Here's how the part is built. I have some questions about the finished solid (model axes, mm). A direction names the side the tool comes from. Round coordinates to 2 decimals unless told otherwise and drop trailing zeros. Order: outer loops, then holes, each group sorted by start corner. A loop starts at its lowest first (then second) coordinate and runs counter-clockwise, first axis right, second up. Notation, with made-up numbers: (-10, 87.25) -> (2, 87.25) arc R33 ccw to (2, 121.25) -> close; hole circle Ø6 at (68, 77). An arc over 180 degrees is marked (long way). Use a Markdown table: item, result. Add a question column.
(1) I want a section at D-D, the plane x = -8. Please give me the cut outline in (y, z), then the cut area to 3 significant figures.
(2) I'm going to push flat-ended pins straight in: P1, Ø12.5, axis at x = 2, z = 16.5, coming from the -Y side; P2, Ø11, axis at x = 1, z = 14.5, coming from the -Y side; P3, Ø5, axis at x = -8, y = -22, coming from the +Z side. Where does each tip first touch, or does it pass through?
(3) I want a section at C-C, the plane z = 13.5. Please give me the cut outline in (x, y).
(4) If I drill on probe 1 along Z at (x, y) = (0, 1.1); probe 2 along Z at (x, y) = (0, 8.55); probe 3 along Y at (x, z) = (8.5, 0.5), over which ranges is the centre line in solid material (lowest first)?
(5) Thinking about a two-plate mould opening in X: for faces 1 (the face through (-12.7, 0.5, -1.8)), 2 (the face through (2, 5.08, 26)), 3 (the face through (0, 10.16, 5)), which applies, pulls with the +X half, pulls with the -X half, needs draft (parallel to the pull), parting line crosses it, or undercut?
(6) I want a section at A-A, the plane z = 27.94. Please give me the cut outline in (x, y), then the cut area to 3 significant figures.
(7) I want a section at B-B, the plane x = 0.5. Please give me the cut outline in (y, z).
(8) On a 3-axis mill with a long thin cutter (end or side, diameter ignored), from which of +Z, -Z, +X, -X, +Y, -Y can I reach the whole of each face in a straight line? I mean faces 4 (the face through (0.18, -34.53, 15.45)), 5 (the face through (2.2, 5.08, 10.5)), 6 (the face through (2.731, 2.504, 32.223)). Say none if no direction works.
from build123d import *

# Parameters (mm, degrees)
F1_DEPTH = 12.7
F2_R     = 2.54
F3_DEPTH = 10.161
F2_R_2   = 5.08
F4_DEPTH = 5.08


with BuildPart() as f1:
    # F0 (on Right) → F1 (new body, symmetric)
    with BuildSketch(Plane.YZ):
        with BuildLine():
            Line((0, 38.1), (0, 0))
            ThreePointArc((0, 0), (-17.78, -17.78), (-35.56, 0))
            ThreePointArc((-35.56, 0), (-34.340603, 6.471077), (-30.849669, 12.054549))
            Line((-30.849669, 12.054549), (-38.318051, 18.942863))
            ThreePointArc((-38.318051, 18.942863), (-43.803804, 10.168836), (-45.72, 0))
            ThreePointArc((-45.72, 0), (-37.536563, -19.756563), (-17.78, -27.94))
            ThreePointArc((-17.78, -27.94), (1.976563, -19.756563), (10.16, 0))
            Line((10.16, 0), (10.16, 38.1))
            Line((10.16, 38.1), (0, 38.1))
        make_face()
        with BuildLine():
            Line((10.16, -27.94), (10.16, 0))
            ThreePointArc((10.16, 0), (1.976563, -19.756563), (-17.78, -27.94))
            Line((-17.78, -27.94), (10.16, -27.94))
        make_face()
    extrude(amount=F1_DEPTH, both=True)

    # F2 (on face) → F3 (cut, through all)
    with BuildSketch(Plane.XZ):
        with Locations((0, 27.94)):
            Circle(F2_R)
        with Locations((0, 12.7)):
            Circle(F2_R)
    extrude(amount=-F3_DEPTH, mode=Mode.SUBTRACT)

    # F2 (on face) → F4 (cut)
    with BuildSketch(Plane.XZ):
        with Locations((0, 27.94)):
            Circle(F2_R_2)
        with Locations((0, 27.94)):
            Circle(F2_R, mode=Mode.SUBTRACT)
        with Locations((0, 12.7)):
            Circle(F2_R_2)
        with Locations((0, 12.7)):
            Circle(F2_R, mode=Mode.SUBTRACT)
    extrude(amount=-F4_DEPTH, mode=Mode.SUBTRACT)


solid = f1.part
Taken from the geometry:
| question | item | result |
|---|---|---|
| 1 | outline | (-45.72, 0) arc R27.94 ccw to (-17.78, -27.94) -> (10.16, -27.94) -> (10.16, 38.1) -> (0, 38.1) -> (0, 0) arc R17.78 cw to (-35.56, 0) arc R17.78 cw to (-30.85, 12.05) -> (-38.32, 18.94) arc R27.94 ccw to start |
| 1 | area | 1,460 mm2 |
| 2 | P1 | stops at y = -43.77 |
| 2 | P2 | stops at y = -44.23 |
| 2 | P3 | stops at z = -16.46 |
| 3 | outline | (-12.7, -42.24) -> (12.7, -42.24) -> (12.7, -32.42) -> (-12.7, -32.42) -> close; (-12.7, 0) -> (-5.02, 0) -> (-5.02, 5.08) -> (-2.41, 5.08) -> (-2.41, 10.16) -> (-12.7, 10.16) -> close; (2.41, 5.08) -> (5.02, 5.08) -> (5.02, 0) -> (12.7, 0) -> (12.7, 10.16) -> (2.41, 10.16) -> close |
| 4 | probe 1 | z = -27.94 to 7.62, 17.78 to 22.86, 33.02 to 38.1 |
| 4 | probe 2 | z = -27.94 to 10.16, 15.24 to 25.4, 30.48 to 38.1 |
| 4 | probe 3 | y = -45.72 to -35.55, 0 to 10.16 |
| 5 | face 1 | pulls with the -X half |
| 5 | face 2 | undercut |
| 5 | face 3 | needs draft |
| 6 | outline | (-12.7, 0) -> (-5.08, 0) -> (-5.08, 5.08) -> (-2.54, 5.08) -> (-2.54, 10.16) -> (-12.7, 10.16) -> close; (2.54, 5.08) -> (5.08, 5.08) -> (5.08, 0) -> (12.7, 0) -> (12.7, 10.16) -> (2.54, 10.16) -> close |
| 6 | area | 181 mm2 |
| 7 | outline | (-45.72, 0) arc R27.94 ccw to (-17.78, -27.94) -> (10.16, -27.94) -> (10.16, 10.21) -> (5.08, 10.21) -> (5.08, 7.64) -> (0, 7.64) -> (0, 0) arc R17.78 cw to (-35.56, 0) arc R17.78 cw to (-30.85, 12.05) -> (-38.32, 18.94) arc R27.94 ccw to start; (0, 17.76) -> (5.08, 17.76) -> (5.08, 15.19) -> (10.16, 15.19) -> (10.16, 25.45) -> (5.08, 25.45) -> (5.08, 22.88) -> (0, 22.88) -> close; (0, 33) -> (5.08, 33) -> (5.08, 30.43) -> (10.16, 30.43) -> (10.16, 38.1) -> (0, 38.1) -> close |
| 8 | face 4 | +Z, +X, -X |
| 8 | face 5 | none |
| 8 | face 6 | -Y |
